from build123d import *

# Parameters (mm, degrees)
EXTRUSION1_DEPTH        = 1.5
ESQUISSE3_W             = 46
ESQUISSE3_H             = 400
EXTRUSION2_DEPTH        = 130
ESQUISSE4_W             = 15
ESQUISSE4_H             = 400
EXTRUSION3_DEPTH        = 145
ESQUISSE7_R             = 3
ENL_V_MAT_EXTRU_1_DEPTH = 20


with BuildPart() as part:
    # Esquisse2 → Extrusion1 (new body)
    with BuildSketch(Plane.ZY.offset(-405.393457589)):
        with BuildLine():
            Line((-30.551651131, -238.253062947), (-30.551651131, -405.753062947))
            Line((-30.551651131, -405.753062947), (-43.551651131, -405.753062947))
            ThreePointArc((-43.551651131, -405.753062947), (-44.965864693, -405.16727651), (-45.551651131, -403.753062947))
            Line((-45.551651131, -403.753062947), (-45.551651131, -393.253062947))
            ThreePointArc((-45.551651131, -393.253062947), (-58.051651131, -380.753062947), (-70.551651131, -393.253062947))
            Line((-70.551651131, -393.253062947), (-70.551651131, -546.503062947))
            ThreePointArc((-70.551651131, -546.503062947), (-58.051651131, -559.003062947), (-45.551651131, -546.503062947))
            Line((-45.551651131, -546.503062947), (-45.551651131, -537.753062947))
            ThreePointArc((-45.551651131, -537.753062947), (-44.965864693, -536.338849385), (-43.551651131, -535.753062947))
            Line((-43.551651131, -535.753062947), (-30.551651131, -535.753062947))
            Line((-30.551651131, -535.753062947), (-30.551651131, -638.253062947))
            Line((-30.551651131, -638.253062947), (-76.551651131, -638.253062947))
            Line((-76.551651131, -638.253062947), (-76.551651131, -238.253062947))
            Line((-76.551651131, -238.253062947), (-30.551651131, -238.253062947))
        make_face()
    extrude(amount=-EXTRUSION1_DEPTH)

    # Esquisse3 → Extrusion2 (add)
    with BuildSketch(Plane.ZY.offset(-405.393457589)):
        with Locations((-53.551651131, -438.253062947)):
            Rectangle(ESQUISSE3_W, ESQUISSE3_H)
    extrude(amount=EXTRUSION2_DEPTH)

    # Esquisse4 → Extrusion3 (add)
    with BuildSketch(Plane.ZY.offset(-275.393457589)):
        with Locations((-84.051651131, -438.253062947)):
            Rectangle(ESQUISSE4_W, ESQUISSE4_H)
    extrude(amount=-EXTRUSION3_DEPTH)

    # Esquisse7 → Enlèv. mat.-Extru.1 (cut)
    with BuildSketch(Plane(origin=(405.393457589, 0, 0), x_dir=(0, 0, -1), z_dir=(1, 0, 0))):
        with Locations((58.051651131, -389.753062947)):
            Circle(ESQUISSE7_R)
        with Locations((58.051651131, -455.753062947)):
            Circle(ESQUISSE7_R)
        with Locations((58.051651131, -549.003062947)):
            Circle(ESQUISSE7_R)
        with BuildLine():
            Line((48.551651131, -414.753062947), (48.551651131, -444.753062947))
            ThreePointArc((48.551651131, -444.753062947), (48.84454435, -445.460169728), (49.551651131, -445.753062947))
            Line((49.551651131, -445.753062947), (63.551651131, -445.753062947))
            ThreePointArc((63.551651131, -445.753062947), (64.258757912, -445.460169728), (64.551651131, -444.753062947))
            Line((64.551651131, -444.753062947), (64.551651131, -414.753062947))
            ThreePointArc((64.551651131, -414.753062947), (64.258757912, -414.045956166), (63.551651131, -413.753062947))
            Line((63.551651131, -413.753062947), (49.551651131, -413.753062947))
            ThreePointArc((49.551651131, -413.753062947), (48.84454435, -414.045956166), (48.551651131, -414.753062947))
        make_face()
        with BuildLine():
            Line((63.551651131, -528.003062947), (63.551651131, -489.003062947))
            ThreePointArc((63.551651131, -489.003062947), (63.258757912, -488.295956166), (62.551651131, -488.003062947))
            Line((62.551651131, -488.003062947), (52.551651131, -488.003062947))
            ThreePointArc((52.551651131, -488.003062947), (51.84454435, -488.295956166), (51.551651131, -489.003062947))
            Line((51.551651131, -489.003062947), (51.551651131, -528.003062947))
            ThreePointArc((51.551651131, -528.003062947), (51.84454435, -528.710169728), (52.551651131, -529.003062947))
            Line((52.551651131, -529.003062947), (62.551651131, -529.003062947))
            ThreePointArc((62.551651131, -529.003062947), (63.258757912, -528.710169728), (63.551651131, -528.003062947))
        make_face()
    extrude(amount=-ENL_V_MAT_EXTRU_1_DEPTH, mode=Mode.SUBTRACT)


solid = part.part
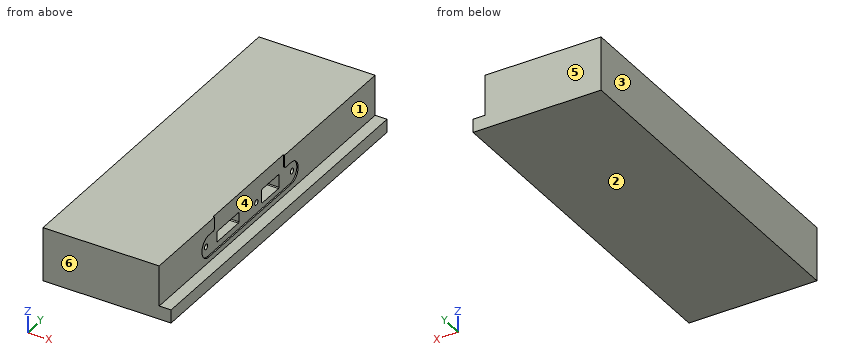
Model file for the job. Use its own axes, mm. Face numbers are marked on the shaded views. A direction names the side the tool comes from. Coordinates: 2 decimals unless noted, no trailing zeros. Loops run counter-clockwise (first coordinate to the right, second up) from the corner with the lowest first, then second, coordinate; pieces in that order, holes last. Notation, with made-up numbers: (-5, 53.25) -> (52, 53.25) arc R16 cw to (52, 82.25) -> close; hole circle Ø10 at (49, 0.5). An arc over 180 degrees is marked (long way). Use one line per item in the form item = value. Start each with the question number.
(1) Pull direction Y, two halves, no side cores. Call the marked faces 3, 4, 5 and 6: pulls with the +Y half, pulls with the -Y half, needs draft (parallel to the pull), parting line crosses it, or undercut.
(2) Cut at A-A on y = -512. Give the cut face in (x, z).
(3) Tool access for the marked faces 1 and 2: list every direction of +Z, -Z, +X, -X, +Y, -Y with a clear straight run to the whole face (end or side of a thin tool).
(4) Probe probe 1 along Y at (x, z) = (385.5, -58.5); probe 2 along X at (y, z) = (-533.5, -66.5); probe 3 along X at (y, z) = (-375.5, -48). List the from-to ranges inside material, lowest first. Write a range as from..to.
(5) Cut at B-B on z = -36. Give the cut face in (x, y).
(6) Flat gauge pins, fed straight in: pin 1 (7 mm diameter, centred on y = -389.75, z = -58.05, fed in from +X); pin 2 (4 mm diameter, centred on x = 405.5, y = -497.5, fed in from +Z); pin 3 (6 mm diameter, centred on y = -503.5, z = -56, fed in from +X). Where does each tip first touch, or does it go through?
(7) Cut at D-D on y = -433. Give the cut face in (x, z), and give its area (3 significant figures).
(8) Cut at C-C on x = 411. Give the cut face in (y, z), and give its area (3 significant figures).
Values:
q1.face_3 = needs draft
q1.face_4 = undercut
q1.face_5 = pulls with the +Y half
q1.face_6 = pulls with the -Y half
q2.outline = (275.39, -91.55) -> (420.39, -91.55) -> (420.39, -76.55) -> (406.89, -76.55) -> (406.89, -70.55) -> (405.39, -70.55) -> (405.39, -63.55) -> (385.39, -63.55) -> (385.39, -51.55) -> (405.39, -51.55) -> (405.39, -30.55) -> (275.39, -30.55) -> close
q3.face_1 = +Z, +X, +Y, -Y
q3.face_2 = -Z, +X, -X, +Y, -Y
q4.probe_1 = -638.25..-551.97, -546.04..-529, -488..-458.72, -452.79..-445.75, -413.75..-392.72, -386.79..-238.25
q4.probe_2 = 275.39..405.39
q4.probe_3 = 275.39..406.89
q5.outline = (275.39, -638.25) -> (406.89, -638.25) -> (406.89, -535.75) -> (405.39, -535.75) -> (405.39, -405.75) -> (406.89, -405.75) -> (406.89, -238.25) -> (275.39, -238.25) -> close
q6.pin_1 = 405.39
q6.pin_2 = -30.55
q6.pin_3 = 385.39
q7.outline = (275.39, -91.55) -> (420.39, -91.55) -> (420.39, -76.55) -> (406.89, -76.55) -> (406.89, -70.55) -> (405.39, -70.55) -> (405.39, -64.55) -> (385.39, -64.55) -> (385.39, -48.55) -> (405.39, -48.55) -> (405.39, -30.55) -> (275.39, -30.55) -> close
q7.area = 7,840 mm2
q8.outline = (-638.25, -91.55) -> (-238.25, -91.55) -> (-238.25, -76.55) -> (-638.25, -76.55) -> close
q8.area = 6,000 mm2
